```python
from build123d import *

# Parameters (mm, degrees)
BOSS_EXTRUDE1_DEPTH = 5
SKETCH2_W           = 14
SKETCH2_H           = 12
CUT_EXTRUDE1_DEPTH  = 116.491341667
SKETCH3_R           = 3.5
SKETCH3_W           = 7
SKETCH3_H           = 24.5
CUT_EXTRUDE2_DEPTH  = 116.491341667
SKETCH4_R           = 1.45
SKETCH4_W           = 8
SKETCH4_H           = 2.9
SKETCH4_W_2         = 2.3
SKETCH4_H_2         = 5.35
SKETCH4_W_3         = 2.9
SKETCH4_H_3         = 8
SKETCH4_W_4         = 5.35
SKETCH4_H_4         = 2.3
CUT_EXTRUDE3_DEPTH  = 116.491341667
SKETCH5_R           = 1.95
CUT_EXTRUDE4_DEPTH  = 116.491341667


with BuildPart() as part:
    # Sketch1 → Boss-Extrude1 (new body)
    with BuildSketch(Plane.XY):
        with BuildLine():
            Line((-83.5, 48), (-83.5, 51))
            Line((-83.5, 51), (-98.5, 51))
            Line((-98.5, 51), (-98.5, 44.95))
            Line((-98.5, 44.95), (-96, 44.95))
            Line((-96, 44.95), (-96, 46.175))
            Line((-96, 46.175), (-93.7, 46.175))
            Line((-93.7, 46.175), (-93.7, 44.95))
            Line((-93.7, 44.95), (-90.5, 44.95))
            Line((-90.5, 44.95), (-90.5, 42.05))
            Line((-90.5, 42.05), (-93.7, 42.05))
            Line((-93.7, 42.05), (-93.7, 40.825))
            Line((-93.7, 40.825), (-96, 40.825))
            Line((-96, 40.825), (-96, 42.05))
            Line((-96, 42.05), (-98.5, 42.05))
            Line((-98.5, 42.05), (-98.5, 36))
            Line((-98.5, 36), (-103.5, 36))
            Line((-103.5, 36), (-103.5, 6))
            Line((-103.5, 6), (-98.5, 6))
            Line((-98.5, 6), (-98.5, -1.55))
            Line((-98.5, -1.55), (-96, -1.55))
            Line((-96, -1.55), (-96, -0.325))
            Line((-96, -0.325), (-93.7, -0.325))
            Line((-93.7, -0.325), (-93.7, -1.55))
            Line((-93.7, -1.55), (-90.5, -1.55))
            Line((-90.5, -1.55), (-90.5, -4.45))
            Line((-90.5, -4.45), (-93.7, -4.45))
            Line((-93.7, -4.45), (-93.7, -5.675))
            Line((-93.7, -5.675), (-96, -5.675))
            Line((-96, -5.675), (-96, -4.45))
            Line((-96, -4.45), (-98.5, -4.45))
            Line((-98.5, -4.45), (-98.5, -9))
            Line((-98.5, -9), (-88.5, -9))
            ThreePointArc((-88.5, -9), (-86.449747468, -4.050252532), (-81.5, -2))
            Line((-81.5, -2), (81.5, -2))
            ThreePointArc((81.5, -2), (86.449747468, -4.050252532), (88.5, -9))
            Line((88.5, -9), (98.5, -9))
            Line((98.5, -9), (98.5, -4.45))
            Line((98.5, -4.45), (96, -4.45))
            Line((96, -4.45), (96, -5.675))
            Line((96, -5.675), (93.7, -5.675))
            Line((93.7, -5.675), (93.7, -4.45))
            Line((93.7, -4.45), (90.5, -4.45))
            Line((90.5, -4.45), (90.5, -1.55))
            Line((90.5, -1.55), (93.7, -1.55))
            Line((93.7, -1.55), (93.7, -0.325))
            Line((93.7, -0.325), (96, -0.325))
            Line((96, -0.325), (96, -1.55))
            Line((96, -1.55), (98.5, -1.55))
            Line((98.5, -1.55), (98.5, 6))
            Line((98.5, 6), (103.5, 6))
            Line((103.5, 6), (103.5, 36))
            Line((103.5, 36), (98.5, 36))
            Line((98.5, 36), (98.5, 42.05))
            Line((98.5, 42.05), (96, 42.05))
            Line((96, 42.05), (96, 40.825))
            Line((96, 40.825), (93.7, 40.825))
            Line((93.7, 40.825), (93.7, 42.05))
            Line((93.7, 42.05), (90.5, 42.05))
            Line((90.5, 42.05), (90.5, 44.95))
            Line((90.5, 44.95), (93.7, 44.95))
            Line((93.7, 44.95), (93.7, 46.175))
            Line((93.7, 46.175), (96, 46.175))
            Line((96, 46.175), (96, 44.95))
            Line((96, 44.95), (98.5, 44.95))
            Line((98.5, 44.95), (98.5, 51))
            Line((98.5, 51), (83.5, 51))
            Line((83.5, 51), (83.5, 48))
            Line((83.5, 48), (69.95, 48))
            Line((69.95, 48), (69.95, 45.5))
            Line((69.95, 45.5), (71.175, 45.5))
            Line((71.175, 45.5), (71.175, 43.2))
            Line((71.175, 43.2), (69.95, 43.2))
            Line((69.95, 43.2), (69.95, 40))
            Line((69.95, 40), (67.05, 40))
            Line((67.05, 40), (67.05, 43.2))
            Line((67.05, 43.2), (65.825, 43.2))
            Line((65.825, 43.2), (65.825, 45.5))
            Line((65.825, 45.5), (67.05, 45.5))
            Line((67.05, 45.5), (67.05, 48))
            Line((67.05, 48), (1.45, 48))
            Line((1.45, 48), (1.45, 45.5))
            Line((1.45, 45.5), (2.675, 45.5))
            Line((2.675, 45.5), (2.675, 43.2))
            Line((2.675, 43.2), (1.45, 43.2))
            Line((1.45, 43.2), (1.45, 40))
            Line((1.45, 40), (-1.45, 40))
            Line((-1.45, 40), (-1.45, 43.2))
            Line((-1.45, 43.2), (-2.675, 43.2))
            Line((-2.675, 43.2), (-2.675, 45.5))
            Line((-2.675, 45.5), (-1.45, 45.5))
            Line((-1.45, 45.5), (-1.45, 48))
            Line((-1.45, 48), (-67.05, 48))
            Line((-67.05, 48), (-67.05, 45.5))
            Line((-67.05, 45.5), (-65.825, 45.5))
            Line((-65.825, 45.5), (-65.825, 43.2))
            Line((-65.825, 43.2), (-67.05, 43.2))
            Line((-67.05, 43.2), (-67.05, 40))
            Line((-67.05, 40), (-69.95, 40))
            Line((-69.95, 40), (-69.95, 43.2))
            Line((-69.95, 43.2), (-71.175, 43.2))
            Line((-71.175, 43.2), (-71.175, 45.5))
            Line((-71.175, 45.5), (-69.95, 45.5))
            Line((-69.95, 45.5), (-69.95, 48))
            Line((-69.95, 48), (-83.5, 48))
        make_face()
    extrude(amount=BOSS_EXTRUDE1_DEPTH)

    # Sketch2 → Cut-Extrude1 (cut, through all)
    with BuildSketch(Plane.XY.offset(5)):
        with Locations((-29.5, 43)):
            Rectangle(SKETCH2_W, SKETCH2_H)
    extrude(amount=-CUT_EXTRUDE1_DEPTH, mode=Mode.SUBTRACT)

    # Sketch3 → Cut-Extrude2 (cut, through all)
    with BuildSketch(Plane.XY.offset(5)):
        with Locations((5, 22.5)):
            Circle(SKETCH3_R)
        with Locations((5, 10.25)):
            Rectangle(SKETCH3_W, SKETCH3_H)
    extrude(amount=-CUT_EXTRUDE2_DEPTH, mode=Mode.SUBTRACT)

    # Sketch4 → Cut-Extrude3 (cut, through all)
    with BuildSketch(Plane.XY.offset(5)):
        with Locations((-101, 23)):
            Circle(SKETCH4_R)
        with Locations(Location((101, 23, 0), (0, 0, 180))):
            Circle(SKETCH4_R)
        with Locations((-94.5, 43.5)):
            Rectangle(SKETCH4_W, SKETCH4_H)
        with Locations((-94.85, 43.5)):
            Rectangle(SKETCH4_W_2, SKETCH4_H_2)
        with Locations((-94.5, -3)):
            Rectangle(SKETCH4_W, SKETCH4_H)
        with Locations((-94.85, -3)):
            Rectangle(SKETCH4_W_2, SKETCH4_H_2)
        with Locations((94.85, -3)):
            Rectangle(SKETCH4_W_2, SKETCH4_H_2)
        with Locations((94.5, -3)):
            Rectangle(SKETCH4_W, SKETCH4_H)
        with Locations((94.85, 43.5)):
            Rectangle(SKETCH4_W_2, SKETCH4_H_2)
        with Locations((94.5, 43.5)):
            Rectangle(SKETCH4_W, SKETCH4_H)
        with Locations((-68.5, 44)):
            Rectangle(SKETCH4_W_3, SKETCH4_H_3)
        with Locations((-68.5, 44.35)):
            Rectangle(SKETCH4_W_4, SKETCH4_H_4)
        with Locations((0, 44)):
            Rectangle(SKETCH4_W_3, SKETCH4_H_3)
        with Locations((0, 44.35)):
            Rectangle(SKETCH4_W_4, SKETCH4_H_4)
        with Locations((68.5, 44.35)):
            Rectangle(SKETCH4_W_4, SKETCH4_H_4)
        with Locations((68.5, 44)):
            Rectangle(SKETCH4_W_3, SKETCH4_H_3)
    extrude(amount=-CUT_EXTRUDE3_DEPTH, mode=Mode.SUBTRACT)

    # Sketch5 → Cut-Extrude4 (cut, through all)
    with BuildSketch(Plane.XY.offset(5)):
        with Locations((-53.5, 9)):
            Circle(SKETCH5_R)
        with Locations((53.5, 9)):
            Circle(SKETCH5_R)
    extrude(amount=-CUT_EXTRUDE4_DEPTH, mode=Mode.SUBTRACT)


solid = part.part
```
Check sheet for the modelled part. Datum: model origin and axes. Units: mm. A direction names the side the tool comes from. Round coordinates to 2 decimals unless told otherwise and drop trailing zeros. Loops run counter-clockwise (first coordinate to the right, second up) from the corner with the lowest first, then second, coordinate; pieces in that order, holes last. Notation, with made-up numbers: (-31.75, 35) - (-22.75, 35) arc R18 cw to (-22.75, 58) - close; hole circle Ø9 at (16.25, -18). An arc over 180 degrees is marked (long way). Answer as a JSON object with one key per item and string values. Group by question number.
Q1. Sectioned sample at C-C, the plane z = 1.5. Count the separate pieces of the cut face and the enclosed holes in it, plus the area to 3 significant figures.
Q2. Sectioned sample at A-A, the plane x = -53.5. Enter the section's corners in (y, z), plus the area to 4 significant figures.
Q3. Gauge pin test, flat ends, axial feed: P1, Ø3, axis at y = 47, z = 3, coming from the -X side; P2, Ø2.5, axis at x = 68.5, z = 2.5, coming from the +Y side; P3, Ø1.1, axis at y = 44, z = 3.5, coming from the -X side. Record the tip position at first contact, or that the pin passes through.
Q4. Set-up check for faces 1 (the face through (98.5, 39, 2)), 2 (the face through (-41, -2, 2)), 3 (the face through (-98.5, 48, 2)), 4 (the face through (-30, 37, 3)): record each of +Z, -Z, +X, -X, +Y, -Y from which the full face is reachable in a straight line by a thin tool's end or side.
Q5. Sectioned sample at D-D, the plane x = -27.5. Enter the section's corners in (y, z), plus the area to 3 significant figures.
Q6. Mould release check, pull along Y, two halves, no side actions. Record for faces 5 (the face through (-94, -9, 2)), 6 (the face through (101, 36, 2)), 7 (the face through (-51.7, 8.25, 2.54)): released by +Y, released by -Y, zero draft, split by the parting line, or undercut.
Q7. Sectioned sample at B-B, the plane y = 9. Enter the section's corners in (x, z).
Q8. Scan lines: line 1 along X through (y, z) = (44, 3.2) (3 decimals); line 2 along Y through (x, z) = (-101, 1.75); line 3 along Y through (x, z) = (94.5, 4.6) (3 decimals). Record each from-to range of solid material in increasing order. Write a range as [from, to].
Solution:
{
 "1": {"separate pieces": "1", "enclosed holes": "4", "area": "9,820 mm²"},
 "2": {"outline": "(-2, 0) - (7.05, 0) - (7.05, 5) - (-2, 5) - close; (10.95, 0) - (48, 0) - (48, 5) - (10.95, 5) - close", "area": "230.5 mm²"},
 "3": {"P1": "stops at x = -98.5", "P2": "stops at y = 40", "P3": "stops at x = -90.5"},
 "4": {"face 1": "+Z, -Z, +X, +Y", "face 2": "+Z, -Z, -Y", "face 3": "+Z, -Z, -X, +Y", "face 4": "+Z, -Z, +Y"},
 "5": {"outline": "(-2, 0) - (37, 0) - (37, 5) - (-2, 5) - close", "area": "195 mm²"},
 "6": {"face 5": "released by -Y", "face 6": "released by +Y", "face 7": "undercut"},
 "7": {"outline": "(-103.5, 0) - (-55.45, 0) - (-55.45, 5) - (-103.5, 5) - close; (-51.55, 0) - (1.5, 0) - (1.5, 5) - (-51.55, 5) - close; (8.5, 0) - (51.55, 0) - (51.55, 5) - (8.5, 5) - close; (55.45, 0) - (103.5, 0) - (103.5, 5) - (55.45, 5) - close"},
 "8": {"line 1": "x = [-90.5, -71.175], [-65.825, -36.5], [-22.5, -2.675], [2.675, 65.825], [71.175, 90.5]", "line 2": "y = [6, 21.55], [24.45, 36]", "line 3": "y = [-9, -5.675], [-0.325, 40.825], [46.175, 51]"}
}
